```python
from build123d import *

# Parameters (mm, degrees)
F0_W      = 9.525
F0_H      = 15.875
F0_W_2    = 6.35
F1_DEPTH  = 17.78
F3_DEPTH  = 17.781
F4_R      = 3.175
F7_R      = 3.2639
F8_DEPTH  = 114.301
F9_R      = 8.89
F10_R     = 8.88999
F11_R     = 1.5875
F11_R_2   = 1.143
F12_DEPTH = 3.175
F15_R     = 1.5875
F15_R_2   = 1.143
F16_DEPTH = 3.175


# Not quite as in the source:
# - two fillets or chamfers of one size are made in one step
# - a fillet or chamfer is up to 0.001 mm smaller than in the source, because OpenCascade refuses the exact size


with BuildPart() as f1:
    # F0 (on Top) → F1 (new body)
    with BuildSketch(Plane.XY):
        Polygon((63.5, 57.15), (-63.5, 57.15), (-63.5, -69.85), (-50.8, -69.85), (-41.275, -69.85), (-3.175, -69.85), (3.175, -69.85), (41.275, -69.85), (50.8, -69.85), (63.5, -69.85), align=None)
        with Locations((-46.0375, -77.7875)):
            Rectangle(F0_W, F0_H)
        with Locations((46.0375, -77.7875)):
            Rectangle(F0_W, F0_H)
        with Locations((0, -77.7875)):
            Rectangle(F0_W_2, F0_H)
    extrude(amount=F1_DEPTH)

    # F2 (on face) → F3 (cut, through all)
    with BuildSketch(Plane.XY.offset(17.78)):
        Polygon((3.175, 50.8), (-58.7375, 50.8), (-58.7375, 25.4), (-52.3875, 25.4), (-52.3875, 19.05), (-58.7375, 19.05), (-58.7375, -31.75), (-52.3875, -31.75), (-52.3875, -38.1), (-58.7375, -38.1), (-58.7375, -63.5), (3.175, -63.5), (58.7375, -63.5), (58.7375, -38.1), (52.3875, -38.1), (52.3875, -31.75), (58.7375, -31.75), (58.7375, 19.05), (52.3875, 19.05), (52.3875, 25.4), (58.7375, 25.4), (58.7375, 50.8), align=None)
    extrude(amount=-F3_DEPTH, mode=Mode.SUBTRACT)

    # F4
    f4_edges = [f1.edges().sort_by_distance(p)[0] for p in [
        (-58.7375, 50.8, 8.89),
        (63.5, 57.15, 8.89),
        (-63.5, 57.15, 8.89),
        (63.5, -69.85, 8.89),
        (-63.5, -69.85, 8.89),
        (50.8, -69.85, 8.89),
        (-50.8, -69.85, 8.89),
        (41.275, -69.85, 8.89),
        (-41.275, -69.85, 8.89),
        (3.175, -69.85, 8.89),
        (-3.175, -69.85, 8.89),
        (58.7375, 25.4, 8.89),
        (58.7375, 50.8, 8.89),
        (-58.7375, 25.4, 8.89),
        (-58.7375, 19.05, 8.89),
        (-58.7375, -31.75, 8.89),
        (-58.7375, -38.1, 8.89),
        (-58.7375, -63.5, 8.89),
        (58.7375, -63.5, 8.89),
        (58.7375, -38.1, 8.89),
        (58.7375, -31.75, 8.89),
        (58.7375, 19.05, 8.89),
    ]]
    fillet(f4_edges, radius=F4_R)

    # F7 (on face) → F8 (cut, through all)
    with BuildSketch(Plane(origin=(-50.8, 0, 0), x_dir=(0, -1, 0), z_dir=(-1, 0, 0))):
        with Locations((77.7875, 9.525)):
            Circle(F7_R)
    extrude(amount=-F8_DEPTH, mode=Mode.SUBTRACT)

    # F9
    f9_edges = [f1.edges().sort_by_distance(p)[0] for p in [
        (-46.0375, -85.725, 17.78),
        (0, -85.725, 17.78),
        (46.0375, -85.725, 17.78),
    ]]
    fillet(f9_edges, radius=F9_R)

    # F10 (radius 8.89 in the source; OpenCascade refuses exactly that, so slightly less here)
    f10_edges = [f1.edges().sort_by_distance(p)[0] for p in [
        (-46.0375, -85.725, 0),
        (0, -85.725, 0),
        (46.0375, -85.725, 0),
    ]]
    fillet(f10_edges, radius=F10_R)

    # F11 (on face) → F12 (cut)
    with BuildSketch(Plane.YZ.offset(63.5)):
        with Locations((-52.07, 8.89)):
            Circle(F11_R)
        with Locations((-46.5709, 8.89)):
            Circle(F11_R_2)
        with Locations((39.37, 8.89)):
            Circle(F11_R)
        with Locations((33.8709, 8.89)):
            Circle(F11_R_2)
        with Locations((-57.5691, 8.89)):
            Circle(F11_R_2)
        with Locations((44.8691, 8.89)):
            Circle(F11_R_2)
    extrude(amount=-F12_DEPTH, mode=Mode.SUBTRACT)

    # F15 (on face) → F16 (cut)
    with BuildSketch(Plane(origin=(-63.5, 0, 0), x_dir=(0, -1, 0), z_dir=(-1, 0, 0))):
        with Locations((-39.37, 8.89)):
            Circle(F15_R)
        with Locations((-33.8709, 8.89)):
            Circle(F15_R_2)
        with Locations((-44.8691, 8.89)):
            Circle(F15_R_2)
        with Locations((52.07, 8.89)):
            Circle(F15_R)
        with Locations((57.5691, 8.89)):
            Circle(F15_R_2)
        with Locations((46.5709, 8.89)):
            Circle(F15_R_2)
    extrude(amount=-F16_DEPTH, mode=Mode.SUBTRACT)


solid = f1.part
```
Geometry check sheet. Reference: the model listing, model coordinates, mm. A direction names the side the tool comes from. Coordinates: 2 decimals unless noted, no trailing zeros. Order: outer loops, then holes, each group sorted by start corner. A loop starts at its lowest first (then second) coordinate and runs counter-clockwise, first axis right, second up. Notation, with made-up numbers: (1, 14) - (35, 14) arc R20 cw to (35, 43) - close; hole circle Ø11 at (-32, 74). An arc over 180 degrees is marked (long way). Use one line per item in the form item = value.
1. Gauge pin test, flat ends, axial feed: pin 1 (1 mm diameter, centred on y = 39, z = 9.5, fed in from +X) (3 decimals); pin 2 (6 mm diameter, centred on x = 5, z = 14, fed in from -Y); pin 3 (7.5 mm diameter, centred on y = -77.79, z = 9.52, fed in from +X). Record the tip position at first contact, or that the pin passes through.
Here are the results:
pin_1 = 60.325
pin_2 = -85.3
pin_3 = 50.8
2. Section check A-A (y = 39.37). Record the boundary of the cut face in (x, z) (1 decimal), then the cut area to 3 significant figures.
Here are the results:
outline = (-63.5, 0) - (-58.7, 0) - (-58.7, 17.8) - (-63.5, 17.8) - (-63.5, 10.5) - (-60.3, 10.5) - (-60.3, 7.3) - (-63.5, 7.3) - close; (58.7, 0) - (63.5, 0) - (63.5, 7.3) - (60.3, 7.3) - (60.3, 10.5) - (63.5, 10.5) - (63.5, 17.8) - (58.7, 17.8) - close
area = 149 mm²
3. Access from +Z, -Z, +X, -X, +Y, -Y to the whole of each face (thin tool, end or side, straight path). Record for faces 1 (the face through (-50.8, -81, 11)), 2 (the face through (-52.388, 22, 9)), 3 (the face through (22, -69.85, 9)), 4 (the face through (-61.935, 40.63, 7.924)), 5 (the face through (60.325, 39, 9)).
Here are the results:
face_1 = +Z, -Z, -X, -Y
face_2 = +Z, -Z
face_3 = +Z, -Z, -Y
face_4 = -X
face_5 = +X
4. Section check B-B (x = -15). Record the boundary of the cut face in (y, z).
Here are the results:
outline = (-69.85, 0) - (-63.5, 0) - (-63.5, 17.78) - (-69.85, 17.78) - close; (50.8, 0) - (57.15, 0) - (57.15, 17.78) - (50.8, 17.78) - close
5. Scan lines: line 1 (X direction, y = -50.5, z = 13); line 2 (Y direction, x = 57, z = 5); line 3 (X direction, y = -35.5, z = 7.5). Record each from-to range of solid material in increasing order.
Here are the results:
line_1 = -63.5 to -58.74, 58.74 to 63.5
line_2 = -69.85 to -63.16, -38.44 to -31.41, 18.71 to 25.74, 50.46 to 57.15
line_3 = -63.5 to -52.39, 52.39 to 63.5
6. Draft check along Z on faces 6 (the face through (1, 57.15, 9)), 7 (the face through (-46.104, -75.197, 7.539)), 8 (the face through (0, -64, 0)). Enter one of: pulls with the +Z half, pulls with the -Z half, needs draft (parallel to the pull), parting line crosses it, or undercut.
Here are the results:
face_6 = needs draft
face_7 = undercut
face_8 = pulls with the -Z half
